Could you check a few things on this model? Use its own coordinates, in mm. Face numbers are marked on the shaded views. A direction names the side the tool comes from. Coordinates: 2 decimals unless noted, no trailing zeros. Order: outer loops, then holes, each group sorted by start corner. A loop starts at its lowest first (then second) coordinate and runs counter-clockwise, first axis right, second up. Notation, with made-up numbers: M 5,-11 L 27,-11 A22 ccw 27,13 Z; hole C 4.5,-35.5 d5. An arc over 180 degrees is marked long. Put each result on its own line as item: value. Start each with the question number.
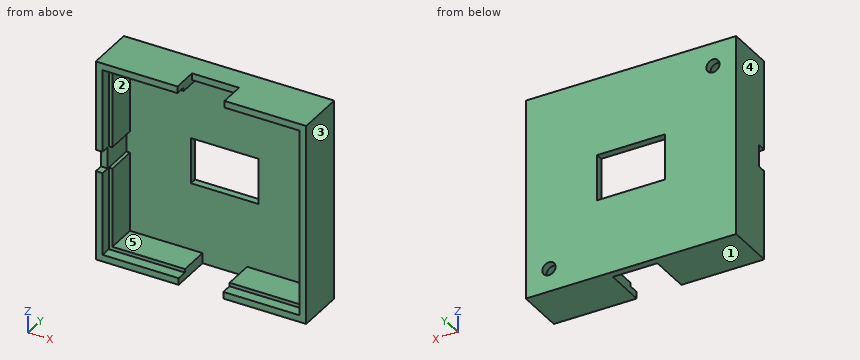
```python
from build123d import *

# Parameters (mm, degrees)
SKETCH1_W           = 59
SKETCH1_H           = 56.5
BOSS_EXTRUDE1_DEPTH = 13.5
SKETCH2_W           = 55.2
SKETCH2_H           = 52.7
CUT_EXTRUDE1_DEPTH  = 11.5
SKETCH10_W          = 19
SKETCH10_H          = 12.9
CUT_EXTRUDE4_DEPTH  = 10
SKETCH11_W          = 6.1
SKETCH11_H          = 2.5
CUT_EXTRUDE5_DEPTH  = 10
SKETCH12_W          = 12.5
SKETCH12_H          = 11.5
CUT_EXTRUDE6_DEPTH  = 10
SKETCH13_W          = 13.2
SKETCH13_H          = 7
CUT_EXTRUDE7_DEPTH  = 10
BOSS_EXTRUDE2_DEPTH = 8.5
SKETCH16_R          = 1.8526
CUT_EXTRUDE8_DEPTH  = 3


with BuildPart() as part:
    # Sketch1 → Boss-Extrude1 (new body)
    with BuildSketch(Plane(origin=(0, 0, 0), x_dir=(1, 0, 0), z_dir=(0, 1, 0))):
        Rectangle(SKETCH1_W, SKETCH1_H)
    extrude(amount=BOSS_EXTRUDE1_DEPTH)

    # Sketch2 → Cut-Extrude1 (cut)
    with BuildSketch(Plane.XZ):
        Rectangle(SKETCH2_W, SKETCH2_H)
    extrude(amount=-CUT_EXTRUDE1_DEPTH, mode=Mode.SUBTRACT)

    # Sketch10 → Cut-Extrude4 (cut)
    with BuildSketch(Plane(origin=(0, 13.5, 0), x_dir=(1, 0, 0), z_dir=(0, 1, 0))):
        Rectangle(SKETCH10_W, SKETCH10_H)
    extrude(amount=-CUT_EXTRUDE4_DEPTH, mode=Mode.SUBTRACT)

    # Sketch11 → Cut-Extrude5 (cut)
    with BuildSketch(Plane.ZY.offset(29.5)):
        with Locations((0, 1.25)):
            Rectangle(SKETCH11_W, SKETCH11_H)
    extrude(amount=-CUT_EXTRUDE5_DEPTH, mode=Mode.SUBTRACT)

    # Sketch12 → Cut-Extrude6 (cut)
    with BuildSketch(Plane(origin=(0, 0, -28.25), x_dir=(-1, 0, 0), z_dir=(0, 0, -1))):
        with Locations((0, 5.75)):
            Rectangle(SKETCH12_W, SKETCH12_H)
    extrude(amount=-CUT_EXTRUDE6_DEPTH, mode=Mode.SUBTRACT)

    # Sketch13 → Cut-Extrude7 (cut)
    with BuildSketch(Plane.XY.offset(28.25)):
        with Locations((0, 3.5)):
            Rectangle(SKETCH13_W, SKETCH13_H)
    extrude(amount=-CUT_EXTRUDE7_DEPTH, mode=Mode.SUBTRACT)

    # Sketch14 → Boss-Extrude2 (add)
    with BuildSketch(Plane.XZ.offset(-11.5)):
        Polygon((-26.6, 25.35), (-26.6, 3.05), (-27.6, 3.05), (-27.6, 26.35), (-6.6, 26.35), (-6.6, 25.35), align=None)
        Polygon((-27.6, -26.35), (-6.25, -26.35), (-6.25, -25.35), (-26.6, -25.35), (-26.6, -3.05), (-27.6, -3.05), align=None)
        Polygon((27.6, 26.35), (27.6, -26.35), (6.25, -26.35), (6.25, -25.35), (26.6, -25.35), (26.6, 25.35), (6.6, 25.35), (6.6, 26.35), align=None)
    extrude(amount=BOSS_EXTRUDE2_DEPTH)

    # Sketch16 → Cut-Extrude8 (cut)
    with BuildSketch(Plane(origin=(0, 13.5, 0), x_dir=(1, 0, 0), z_dir=(0, 1, 0))):
        with Locations(Location((23, 21.75, 0), (0, 0, 90))):
            Circle(SKETCH16_R)
        with Locations(Location((-23, -21.75, 0), (0, 0, 90))):
            Circle(SKETCH16_R)
    extrude(amount=-CUT_EXTRUDE8_DEPTH, mode=Mode.SUBTRACT)


solid = part.part
```
Item 1: If we section it at C-C on y = 4.25: Write out the boundary of the cut face in (x, z).
Item 2: If we section it at B-B on x = 0: Write out the boundary of the cut face in (y, z).
Item 3: For the marked faces 1 and 2, which set-ups out of +Z, -Z, +X, -X, +Y, -Y let a thin tool reach every point of the face, with its end or its side?
Item 4: If we section it at A-A on z = -5: Write out the boundary of the cut face in (x, y), then the cut area to 3 significant figures.
Item 5: I need wall thicknesses on probe 1 along X at (y, z) = (6.75, -3); probe 2 along Z at (x, y) = (-17, 6.25); probe 3 along X at (y, z) = (2.5, 13). Which ranges of each line are inside material? Lowest first, please.
Item 6: If we section it at D-D on z = 9.5: Write out the boundary of the cut face in (x, y).
Item 7: If we mould it in two halves opening along X, with no side actions, what happens to the marked faces 3, 4 and 5? For each: released by +X, released by -X, zero draft, split by the parting line, or undercut.
Item 8: For pin 1 Ø3 at (x, z) = (-15.5, -5.5) entering from -Y; pin 2 Ø5 at (x, y) = (0, 9.5) entering from -Z; pin 3 Ø2 at (x, z) = (0.5, 27.5) entering from -Y, each with a flat end and sliding along its axis, tell me the tip position at first contact or that it passes through.
Geometry check:
1. outline: M -29.5,-28.25 L -6.25,-28.25 L -6.25,-25.35 L -26.6,-25.35 L -26.6,-3.05 L -27.6,-3.05 L -27.6,3.05 L -26.6,3.05 L -26.6,25.35 L -6.6,25.35 L -6.6,28.25 L -29.5,28.25 Z; M 6.25,-28.25 L 29.5,-28.25 L 29.5,28.25 L 6.6,28.25 L 6.6,25.35 L 26.6,25.35 L 26.6,-25.35 L 6.25,-25.35 Z
2. outline: M 7,26.35 L 11.5,26.35 L 11.5,6.45 L 13.5,6.45 L 13.5,28.25 L 7,28.25 Z; M 11.5,-28.25 L 13.5,-28.25 L 13.5,-6.45 L 11.5,-6.45 Z
3. face 1: -Z, +X, -X, +Y, -Y
3. face 2: -Y
4. outline: M -29.5,0 L -27.6,0 L -27.6,3 L -26.6,3 L -26.6,11.5 L -9.5,11.5 L -9.5,13.5 L -29.5,13.5 Z; M 9.5,11.5 L 26.6,11.5 L 26.6,3 L 27.6,3 L 27.6,0 L 29.5,0 L 29.5,13.5 L 9.5,13.5 Z
4. area: 141 mm²
5. probe 1: x = -29.5 to -27.6, 26.6 to 29.5
5. probe 2: z = -28.25 to -25.35, 25.35 to 28.25
5. probe 3: x = -29.5 to -27.6, 27.6 to 29.5
6. outline: M -29.5,0 L -27.6,0 L -27.6,3 L -26.6,3 L -26.6,11.5 L 26.6,11.5 L 26.6,3 L 27.6,3 L 27.6,0 L 29.5,0 L 29.5,13.5 L -29.5,13.5 Z
7. face 3: released by +X
7. face 4: released by -X
7. face 5: undercut
8. pin 1: stops at y = 11.5
8. pin 2: stops at z = -28.25
8. pin 3: stops at y = 7
